Geometry: final body of the model. Coordinates: model frame, mm. A direction names the side the tool comes from. Round coordinates to 2 decimals unless told otherwise and drop trailing zeros. Loops run counter-clockwise (first coordinate to the right, second up) from the corner with the lowest first, then second, coordinate; pieces in that order, holes last. Notation, with made-up numbers: M -6,-30 L 27,-30 A12 ccw 27,-17 Z; hole C -24.75,2 d1. An arc over 180 degrees is marked long. Answer as a JSON object with one key per item and string values.
from build123d import *

# Parameters (mm, degrees)
SKETCH1_R           = 7.5
BOSS_EXTRUDE1_DEPTH = 15
BOSS_EXTRUDE2_DEPTH = 42
CHAMFER2_SIZE       = 15
SKETCH4_W           = 18.864791466
SKETCH4_H           = 20
CUT_EXTRUDE2_DEPTH  = 10


with BuildPart() as part:
    # Sketch1 → Boss-Extrude1 (new body)
    with BuildSketch(Plane(origin=(0, 0, 0), x_dir=(1, 0, 0), z_dir=(0, 1, 0))):
        with BuildLine():
            Line((-133.396551724, -75), (0, -75))
            Line((0, -75), (0, 0))
            Line((0, 0), (-150, 0))
            Line((-150, 0), (-150, -58.396551724))
            ThreePointArc((-150, -58.396551724), (-145.136962591, -70.136962591), (-133.396551724, -75))
        make_face()
        with Locations(Location((-133.396551724, -58.396551724, 0), (0, 0, 270))):
            Circle(SKETCH1_R, mode=Mode.SUBTRACT)
    extrude(amount=BOSS_EXTRUDE1_DEPTH)

    # Sketch3 → Boss-Extrude2 (add)
    with BuildSketch(Plane(origin=(0, 15, 0), x_dir=(1, 0, 0), z_dir=(0, 1, 0))):
        Polygon((0, 0), (-150, 0), (-150, -15.113333235), (-18.864791466, -15.113333235), (-18.864791466, -75), (0, -75), (0, -15.113333235), align=None)
    extrude(amount=BOSS_EXTRUDE2_DEPTH)

    # Chamfer2
    chamfer2_edges = [part.edges().sort_by_distance(p)[0] for p in [
        (-150, 57, 7.556666618),
    ]]
    chamfer(chamfer2_edges, length=CHAMFER2_SIZE)

    # Sketch4 → Cut-Extrude2 (cut)
    with BuildSketch(Plane(origin=(0, 57, 0), x_dir=(1, 0, 0), z_dir=(0, 1, 0))):
        with Locations((-9.432395733, -45.113333235)):
            Rectangle(SKETCH4_W, SKETCH4_H)
    extrude(amount=-CUT_EXTRUDE2_DEPTH, mode=Mode.SUBTRACT)


solid = part.part
1) Section query A-A (z = 63.5). Return the cut outline in (x, y), and give its area (3 significant figures).
Results:
{"outline": "M -149.2,0 L -138.89,0 L -138.89,15 L -149.2,15 Z; M -127.9,0 L 0,0 L 0,57 L -18.86,57 L -18.86,15 L -127.9,15 Z", "area": "2,870 mm2"}
2) Section query C-C (x = -60). Return the cut outline in (y, z).
Results:
{"outline": "M 0,0 L 57,0 L 57,15.11 L 15,15.11 L 15,75 L 0,75 Z"}
3) Reachability of faces 4 (the flat face through (-85, 15, 45)), 5 (the flat face through (-10, 52, 55.113)), 6 (the flat face through (-10, 57, 65)) from +Z, -Z, +X, -X, +Y, -Y: full face, straight path, thin tool, end or side. Return the list, or none.
Results:
{"face 4": "+Z, -X, +Y", "face 5": "+X, -X, +Y", "face 6": "+Z, -Z, +X, -X, +Y"}
4) Section query D-D (y = 11.5). Return the cut outline in (x, z).
Results:
{"outline": "M -150,0 L 0,0 L 0,75 L -133.4,75 A16.6 ccw -150,58.4 Z; hole C -133.4,58.4 d15"}
5) Ray query, line 1 (X direction, y = 48.5, z = 69.5); line 2 (Z direction, x = -53.5, y = 40); line 3 (Y direction, x = -41, z = 25). Return the intervals inside material, ascending.
Results:
{"line 1": "-18.86 to 0", "line 2": "0 to 15.11", "line 3": "0 to 15"}
6) Pin query (flat end, axial travel): P1, Ø4, axis at x = -131, z = 18.5, coming from the +Y side; P2, Ø15, axis at x = -10.5, z = 43, coming from the +Y side; P3, Ø12.5, axis at x = -102, y = 43, coming from the +Z side. Return the tip coordinate at first contact, or that it passes through.
Results:
{"P1": "y = 15", "P2": "y = 47", "P3": "z = 15.11"}
7) Pull-direction query (Z, two-part tool) for faces 1 (the flat face through (0, 28, 38)), 2 (the flat face through (-10, 47, 45)), 3 (the flat face through (-74, 28, 0)); classes: +Z half, -Z half, draft (parallel to the pull), parting line (faces both ways), or undercut.
Results:
{"face 1": "draft", "face 2": "undercut", "face 3": "-Z half"}
8) Section query B-B (y = 21). Return the cut outline in (x, z).
Results:
{"outline": "M -150,0 L 0,0 L 0,75 L -18.86,75 L -18.86,15.11 L -150,15.11 Z"}
